```python
from build123d import *

# Parameters (mm, degrees)
EXTRUDE_1_DEPTH          = 9.5
SKETCH_3_R               = 9
CUT_EXTRUDE_1_DEPTH      = 10
SWEEP_1_PITCH            = 4
CHAMFER_1_SIZE           = 1
CUT_EXTRUDE_3_DEPTH      = 0.4
SKETCH_12_R              = 2.5
CUT_EXTRUDE_4_DEPTH      = 0.4
CUT_EXTRUDE_6_DEPTH      = 32.468328554
CUT_EXTRUDE_6_DEPTH_BACK = 0.4
SKETCH_11_W              = 5
SKETCH_11_H              = 5
CUT_EXTRUDE_7_DEPTH      = 0.4


with BuildPart() as part:
    # 草图1 → 凸台-拉伸1 (new body)
    with BuildSketch(Plane.XY):
        Polygon((15, 0), (7.5, 12.990381057), (-7.5, 12.990381057), (-15, 0), (-7.5, -12.990381057), (7.5, -12.990381057), align=None)
    extrude(amount=EXTRUDE_1_DEPTH)

    # 草图3 → 切除-拉伸1 (cut)
    with BuildSketch(Plane(origin=(0, 0, 0), x_dir=(-1, 0, 0), z_dir=(0, 0, -1))):
        Circle(SKETCH_3_R)
    extrude(amount=-CUT_EXTRUDE_1_DEPTH, mode=Mode.SUBTRACT)

    # 扫描1: the profile of 草图5 profile screwed along a right-hand helix of 1.5 turns, 12 arcs to a turn; built about Z, then put on its axis
    sweep_1_z = Axis((0, 0, 0), (0, 0, 1))
    sweep_1_corners = [(9.0003, 0, -1.7503), (9.0003, 0, 1.7503), (7.5, 0, 0.25), (7.5, 0, -0.25)]
    with BuildLine(mode=Mode.PRIVATE) as sweep_1_profile:
        Line(sweep_1_corners[0], sweep_1_corners[1])
        Line(sweep_1_corners[1], sweep_1_corners[2])
        Line(sweep_1_corners[2], sweep_1_corners[3])
        Line(sweep_1_corners[3], sweep_1_corners[0])
    sweep_1_cap = Face(sweep_1_profile.wire())
    sweep_1_turn_angles = [0, 15, 30, 45, 60, 75, 90, 105, 120, 135, 150, 165, 180, 195, 210, 225, 240, 255, 270, 285, 300, 315, 330, 345, 360]
    sweep_1_turn_weights = [1, 0.9659258262890683, 1, 0.9659258262890683, 1, 0.9659258262890683, 1, 0.9659258262890683, 1, 0.9659258262890683, 1, 0.9659258262890683, 1, 0.9659258262890683, 1, 0.9659258262890683, 1, 0.9659258262890683, 1, 0.9659258262890683, 1, 0.9659258262890683, 1, 0.9659258262890683, 1]
    sweep_1_turn_rails = [Edge.make_bspline([Vector(p[0], p[1], 0).rotate(sweep_1_z, sweep_1_turn_angles[k]) / sweep_1_turn_weights[k] + Vector(0, 0, p[2] + SWEEP_1_PITCH * sweep_1_turn_angles[k] / 360) for k in range(25)], [0, 0, 0, 1, 1, 2, 2, 3, 3, 4, 4, 5, 5, 6, 6, 7, 7, 8, 8, 9, 9, 10, 10, 11, 11, 12, 12, 12], 2, sweep_1_turn_weights) for p in sweep_1_corners]
    sweep_1_turn_sides = [Face.make_surface_from_curves(sweep_1_turn_rails[p[0]], sweep_1_turn_rails[p[1]]) for p in [(0, 1), (1, 2), (2, 3), (3, 0)]]
    sweep_1_last_angles = [360, 375, 390, 405, 420, 435, 450, 465, 480, 495, 510, 525, 540]
    sweep_1_last_weights = [1, 0.9659258262890683, 1, 0.9659258262890683, 1, 0.9659258262890683, 1, 0.9659258262890683, 1, 0.9659258262890683, 1, 0.9659258262890658, 1]
    sweep_1_last_rails = [Edge.make_bspline([Vector(p[0], p[1], 0).rotate(sweep_1_z, sweep_1_last_angles[k]) / sweep_1_last_weights[k] + Vector(0, 0, p[2] + SWEEP_1_PITCH * sweep_1_last_angles[k] / 360) for k in range(13)], [0, 0, 0, 1, 1, 2, 2, 3, 3, 4, 4, 5, 5, 6, 6, 6], 2, sweep_1_last_weights) for p in sweep_1_corners]
    sweep_1_last_sides = [Face.make_surface_from_curves(sweep_1_last_rails[p[0]], sweep_1_last_rails[p[1]]) for p in [(0, 1), (1, 2), (2, 3), (3, 0)]]
    sweep_1 = Plane(origin=(0, 0, 1.75), x_dir=(1, 0, 0), z_dir=(0, 0, 1)) * Solid(Shell([*sweep_1_turn_sides, *sweep_1_last_sides, sweep_1_cap, sweep_1_cap.rotate(sweep_1_z, 540).moved(Location((0, 0, SWEEP_1_PITCH * 540 / 360)))]))
    add(sweep_1)

    # 倒角1
    chamfer_1_edges = [part.edges().sort_by_distance(p)[0] for p in [
        (-11.25, 6.495190528, 9.5),
        (-11.25, -6.495190528, 9.5),
        (0, -12.990381057, 9.5),
        (11.25, -6.495190528, 9.5),
        (11.25, 6.495190528, 9.5),
        (11.25, -6.495190528, 0),
        (0, -12.990381057, 0),
        (-11.25, -6.495190528, 0),
        (-11.25, 6.495190528, 0),
        (0, 12.990381057, 0),
        (11.25, 6.495190528, 0),
        (0, 12.990381057, 9.5),
    ]]
    chamfer(chamfer_1_edges, length=CHAMFER_1_SIZE)

    # 草图7 → 切除-拉伸3 (cut)
    with BuildSketch(Plane(origin=(11.25, 6.495190528, 0), x_dir=(0, 0, -1), z_dir=(0.8660254037844386, 0.5000000000000003, 0))):
        Polygon((-2.25, 2.886751346), (-7.25, 0), (-2.25, -2.886751346), align=None)
    extrude(amount=-CUT_EXTRUDE_3_DEPTH, mode=Mode.SUBTRACT)

    # 草图12 → 切除-拉伸4 (cut)
    with BuildSketch(Plane(origin=(-11.25, 6.495190528, 0), x_dir=(0, 0, 1), z_dir=(-0.8660254037844384, 0.5000000000000006, 0))):
        with Locations(Location((4.75, 0, 0), (0, 0, 270))):
            Circle(SKETCH_12_R)
    extrude(amount=-CUT_EXTRUDE_4_DEPTH, mode=Mode.SUBTRACT)

    # 草图10 → 切除-拉伸6 (cut, two sides: drawn at the far end of the back side and taken through both)
    with BuildSketch(Plane(origin=(0, 12.990381057, 0), x_dir=(1, 0, 0), z_dir=(0, 1, 0)).offset(-CUT_EXTRUDE_6_DEPTH_BACK)):
        Polygon((2.075735931, -2.25), (-2.5, -6.825735931), (-2.075735931, -7.25), (2.5, -2.674264069), align=None)
        Polygon((-2.5, -2.674264069), (2.075735931, -7.25), (2.5, -6.825735931), (-2.075735931, -2.25), align=None)
    extrude(amount=CUT_EXTRUDE_6_DEPTH + CUT_EXTRUDE_6_DEPTH_BACK, mode=Mode.SUBTRACT)

    # 草图11 → 切除-拉伸7 (cut)
    with BuildSketch(Plane(origin=(11.25, -6.495190528, 0), x_dir=(0, 0, -1), z_dir=(0.8660254037844387, -0.5000000000000001, 0))):
        with Locations((-4.75, 0)):
            Rectangle(SKETCH_11_W, SKETCH_11_H)
    extrude(amount=-CUT_EXTRUDE_7_DEPTH, mode=Mode.SUBTRACT)


solid = part.part
```
Design review of the part built by this model. Coordinates are the model's own, in mm. A direction names the side the tool comes from. Give positions to 0.01 mm unless a question says otherwise; leave off trailing zeros. Return JSON: item names as keys, results as strings. Group by question number.
(1) Machinability: for faces 1 (the flat face through (11.198, -6.586, 1.364)), 2 (the flat face through (8, 0, 2)), 3 (the flat face through (-1.477, 12.788, 3.698)), which of the approach directions +Z, -Z, +X, -X, +Y, -Y give a long, thin tool a straight path to every point of the face, cutting with its end or side? Answer none if there is none.
(2) To check wall thickness, follow probe 1 along Y at (x, z) = (0, 6.55); probe 2 along Y at (x, z) = (0, 2); probe 3 along X at (y, z) = (5, 4.5). State the ranges of each line that lie inside material, in increasing order.
(3) Insertion check: pin 1 (0.5 mm diameter, centred on x = 8, z = 1.5, fed in from -Y); pin 2 (12 mm diameter, centred on x = 1.5, y = -2.5, fed in from +Z); pin 3 (11 mm diameter, centred on x = 0, y = 0, fed in from -Z); pin 4 (0.5 mm diameter, centred on x = -8.5, z = 7.5, fed in from -Y). Each pin has a flat end and moves straight along its axis. Give the tip position at first contact, or say it passes through.
(4) Mouldability with a two-part tool opening along Z and no side actions: class faces 4 (the flat face through (0.1, 12.5, 0.51)), 5 (the flat face through (9, -2, 9.5)), 6 (the flat face through (11.1, -6.4, 2.25)), 7 (the flat face through (10.35, 7.66, 4.72)) as +Z half, -Z half, draft (parallel to the pull), parting line (faces both ways), or undercut.
Reported:
{
 "1": {"face 1": "+Z, -Z, +X, -Y", "face 2": "-Z", "face 3": "+Y"},
 "2": {"probe 1": "y = -12.99 to -9, 7.5 to 12.99", "probe 2": "y = -12.99 to -9, 8 to 12.99", "probe 3": "x = -11.65 to -6.76, 7.34 to 11.65, 11.84 to 12.11"},
 "3": {"pin 1": "stops at y = -12.56", "pin 2": "stops at z = 6.81", "pin 3": "passes through", "pin 4": "stops at y = -11.69"},
 "4": {"face 4": "-Z half", "face 5": "+Z half", "face 6": "undercut", "face 7": "undercut"}
}
